Check sheet for the modelled part. Datum: model origin and axes. Units: mm. Coordinates: 2 decimals unless noted, no trailing zeros. Loops run counter-clockwise (first coordinate to the right, second up) from the corner with the lowest first, then second, coordinate; pieces in that order, holes last. Notation, with made-up numbers: M 19.25,-36.5 L 57.25,-36.5 A19 ccw 57.25,0.5 Z; hole C 73,85.25 d8. An arc over 180 degrees is marked long. Return JSON: item names as keys, results as strings.
from build123d import *

# Parameters (mm, degrees)
CROQUIS1_R              = 1.3
SALIENTE_EXTRUIR1_DEPTH = 3


with BuildPart() as part:
    # Croquis1 → Saliente-Extruir1 (new body)
    with BuildSketch(Plane(origin=(0, 0, 0), x_dir=(1, 0, 0), z_dir=(0, 1, 0))):
        Polygon((17, 33.65), (30.865, 33.65), (39.365, 33.65), (53.23, 33.65), (53.23, 30.65), (61.73, 30.65), (61.73, 33.65), (70.23, 33.65), (70.23, 31.85), (67.23, 31.85), (67.23, 26.85), (70.23, 26.85), (70.23, 6.8), (67.23, 6.8), (67.23, 1.8), (70.23, 1.8), (70.23, 0), (61.73, 0), (61.73, 3), (53.23, 3), (53.23, 0), (39.365, 0), (39.365, 3), (30.865, 3), (30.865, 0), (17, 0), (17, 3), (8.5, 3), (8.5, 0), (0, 0), (0, 1.8), (3, 1.8), (3, 6.8), (0, 6.8), (0, 26.85), (3, 26.85), (3, 31.85), (0, 31.85), (0, 33.65), (8.5, 33.65), (8.5, 30.65), (17, 30.65), align=None)
        with Locations(Location((7.3, 26.35, 0), (0, 0, 270))):
            Circle(CROQUIS1_R, mode=Mode.SUBTRACT)
        with Locations(Location((7.3, 7.3, 0), (0, 0, 270))):
            Circle(CROQUIS1_R, mode=Mode.SUBTRACT)
        with Locations(Location((62.93, 26.35, 0), (0, 0, 270))):
            Circle(CROQUIS1_R, mode=Mode.SUBTRACT)
        with Locations(Location((62.93, 7.3, 0), (0, 0, 270))):
            Circle(CROQUIS1_R, mode=Mode.SUBTRACT)
    extrude(amount=SALIENTE_EXTRUIR1_DEPTH)


solid = part.part
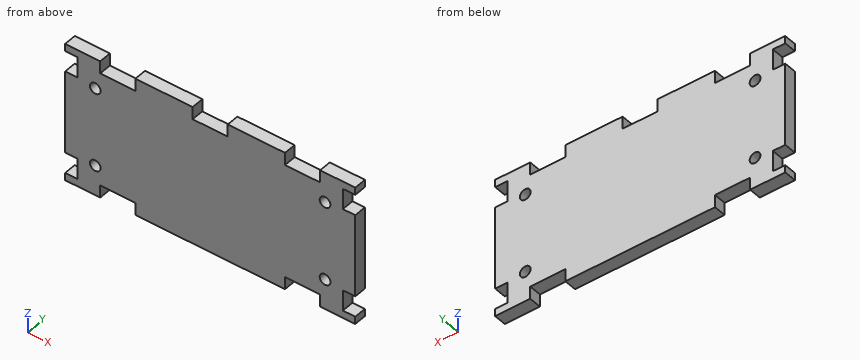
1) Section check B-B on y = 1. Count the separate pieces of the cut face and the enclosed holes in it, then the cut area to 3 significant figures.
Answers:
{"separate pieces": "1", "enclosed holes": "4", "area": "2,150 mm²"}
2) Section check C-C on z = -29.5. Record the cut outline in (x, y).
Answers:
{"outline": "M 3,0 L 67.23,0 L 67.23,3 L 3,3 Z"}
3) Scan lines: line 1 along X through (y, z) = (0.6, -7.5); line 2 along Z through (x, y) = (38.5, 0.8); line 3 along X through (y, z) = (2.85, -30.5). Record each from-to range of solid material in increasing order. Write a range as [from, to].
Answers:
{"line 1": "[0, 6.02], [8.58, 61.65], [64.21, 70.23]", "line 2": "[-33.65, -3]", "line 3": "[3, 67.23]"}
4) Go/stop test with a flat-tipped pin: pin 1 Ø1 at (x, y) = (14.5, 1) entering from -Z. Record where the tip stops, or that it passes through.
Answers:
{"pin 1": "z = -30.65"}
5) Section check A-A on x = 7.3. Record the cut outline in (y, z).
Answers:
{"outline": "M 0,-33.65 L 3,-33.65 L 3,-27.65 L 0,-27.65 Z; M 0,-25.05 L 3,-25.05 L 3,-8.6 L 0,-8.6 Z; M 0,-6 L 3,-6 L 3,0 L 0,0 Z"}
